Autodesk Inventor part; units mm, degrees
ref_plane "YZ Plane" through (0, 0, 0) normal (1, 0, 0) x (0, 1, 0)
ref_plane "XZ Plane" through (0, 0, 0) normal (0, 1, 0) x (-1, 0, 0)
ref_plane "XY Plane" through (0, 0, 0) normal (0, 0, 1) x (1, 0, 0)
sketch "Sketch1" plane through (0, 0, 0) normal (0, 0, 1) x (1, 0, 0)
  line L0 (-175, -50) -> (175, -50)
  line L1 (175, -50) -> (175, 50)
  line L2 (175, 50) -> (-175, 50)
  line L3 (-175, 50) -> (-175, -50)
  line L4 (-175, -50) -> (175, 50) construction
  line L5 (175, -50) -> (-175, 50) construction
  point P0 (0, 0)
  dimension "d0" = 350
  dimension "d1" = 100
extrude "Extrusion1" add sketch "Sketch1" along normal blind 180
sketch "Sketch2" plane through (-175, -50, 0) normal (-1, 0, 0) x (0, 0, 1)
  line L0 (180, 0) -> (180, 100)
  line L1 (180, 100) -> (0, 0)
  line L2 (0, 0) -> (196.9773, -61.362)
  line L3 (196.9773, -61.362) -> (180, 100)
  point P0 (0, 50)
extrude "Extrusion2" cut sketch "Sketch2" against normal through all
sketch "Sketch3" plane through (0, 0, 0) normal (0, 0, -1) x (-1, 0, 0)
  circle A0 centre (150, 0) radius 5
  line L0 (-175, 50) -> (175, 50)
  line L1 (175, -50) -> (-175, -50)
  circle A1 centre (-150, 0) radius 5
  point P0 (0, 0)
  dimension "d8" = 10
extrude "Extrusion3" cut sketch "Sketch3" against normal through all
properties part number "Banco"
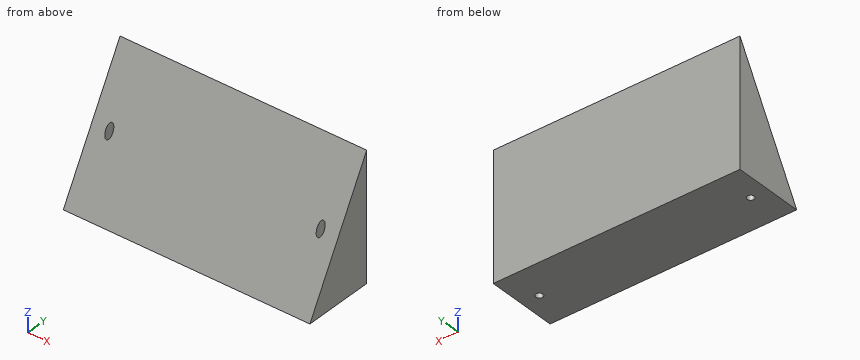
Part model, mm, in its own coordinate system. Give positions to 0.01 mm unless a question says otherwise; leave off trailing zeros. Write each loop counter-clockwise with the first axis right and the second up, starting at its lowest first coordinate (ties: lowest second). Pieces come first, ordered by that corner, then holes. Notation, with made-up numbers: M 8,62.5 L 46,62.5 A23 ccw 46,84.5 Z; hole C 35.25,76 d7. An arc over 180 degrees is marked long. Use CSV: the item, a comma, the result in double quotes.
Item 1: Pin check, flat tips, straight feed: P1, Ø11.5, axis at x = -150, y = 0, coming from the +Z side; P2, Ø2, axis at x = 114.5, y = 37, coming from the +Z side; P3, Ø12, axis at x = -48.5, z = 56, coming from the -Y side. Stop position of each tip, or through.
Taken from the geometry:
P1,"stops at z = 100.35"
P2,"stops at z = 158.4"
P3,"stops at y = -22.22"
Item 2: Slice it at D-D on x = -133. Write the cut outline in (y, z), plus the area to 3 significant figures.
Taken from the geometry:
outline,"M -50,0 L 50,0 L 50,180 Z"
area,"9,000 mm²"
Item 3: Slice it at A-A on y = 0. Write the cut outline in (x, z).
Taken from the geometry:
outline,"M -175,0 L -155,0 L -155,90 L -175,90 Z; M -145,0 L 145,0 L 145,90 L -145,90 Z; M 155,0 L 175,0 L 175,90 L 155,90 Z"
Item 4: Slice it at C-C on z = 72. Write the cut outline in (x, y), plus the area to 3 significant figures.
Taken from the geometry:
outline,"M -175,-10 L 175,-10 L 175,50 L -175,50 Z; hole C -150,0 d10; hole C 150,0 d10"
area,"20,800 mm²"
Item 5: Slice it at B-B on x = 150. Write the cut outline in (y, z), plus the area to 3 significant figures.
Taken from the geometry:
outline,"M -50,0 L -5,0 L -5,81 Z; M 5,0 L 50,0 L 50,180 L 5,99 Z"
area,"8,100 mm²"
Item 6: Drill centre lines: probe 1 along X at (y, z) = (0, 52); probe 2 along Y at (x, z) = (150, 47); probe 3 along Y at (x, z) = (150, 27.5). Where is each one in solid material? Low to high.
Taken from the geometry:
probe 1,"x = -175 to -155, -145 to 145, 155 to 175"
probe 2,"y = -23.89 to -5, 5 to 50"
probe 3,"y = -34.72 to -5, 5 to 50"
